from build123d import *

# Parameters (mm, degrees)
F0_W      = 498.475
F0_H      = 254
F1_DEPTH  = 36.576
F2_W      = 577.8754
F2_H      = 333.502
F3_DEPTH  = 3.175
F4_W      = 76.2
F4_H      = 114.3
F5_DEPTH  = 3.175
F6_W      = 76.2
F6_H      = 228.6
F7_DEPTH  = 3.175
F8_W      = 25.4
F8_H      = 152.4
F9_DEPTH  = 6.35
F10_W     = 25.4
F10_H     = 152.4
F11_DEPTH = 6.35
F12_W     = 571.5
F12_H     = 92.075
F13_DEPTH = 3.175
F14_W     = 508
F14_H     = 25.4
F15_DEPTH = 6.35


with BuildPart() as f1:
    # F0 (on Front) → F1 (new body)
    with BuildSketch(Plane.XZ):
        Rectangle(F0_W, F0_H)
    extrude(amount=F1_DEPTH)

    # F2 (on face) → F3 (join)
    with BuildSketch(Plane.XZ.offset(36.576)):
        Rectangle(F2_W, F2_H)
    extrude(amount=F3_DEPTH)

    # F4 (on face) → F5 (join)
    with BuildSketch(Plane.YZ.offset(288.9377)):
        with Locations((-1.651, 57.15)):
            Rectangle(F4_W, F4_H)
        with Locations((-1.651, -57.15)):
            Rectangle(F4_W, F4_H)
    extrude(amount=F5_DEPTH)

    # F6 (on face) → F7 (join)
    with BuildSketch(Plane(origin=(-288.9377, 0, 0), x_dir=(0, -1, 0), z_dir=(-1, 0, 0))):
        with Locations((1.651, 0)):
            Rectangle(F6_W, F6_H)
    extrude(amount=F7_DEPTH)

    # F8 (on face) → F9 (join)
    with BuildSketch(Plane.YZ.offset(-288.9377)):
        with Locations((-1.651, 0)):
            Rectangle(F8_W, F8_H)
    extrude(amount=F9_DEPTH)

    # F10 (on face) → F11 (join)
    with BuildSketch(Plane(origin=(288.9377, 0, 0), x_dir=(0, -1, 0), z_dir=(-1, 0, 0))):
        with Locations((1.651, 0)):
            Rectangle(F10_W, F10_H)
    extrude(amount=F11_DEPTH)

    # F12 (on face) → F13 (join)
    with BuildSketch(Plane.XY.offset(166.751)):
        with Locations((0, 6.2865)):
            Rectangle(F12_W, F12_H)
    extrude(amount=F13_DEPTH)

    # F14 (on face) → F15 (join)
    with BuildSketch(Plane(origin=(0, 0, 166.751), x_dir=(1, 0, 0), z_dir=(0, 0, -1))):
        with Locations((0, -26.924)):
            Rectangle(F14_W, F14_H)
    extrude(amount=F15_DEPTH)


solid = f1.part
Source: CAD feature listing. Evaluate the final solid. Frame: model axes, mm. A direction names the side the tool comes from. Coordinates: 2 decimals unless noted, no trailing zeros. Order: outer loops, then holes, each group sorted by start corner. A loop starts at its lowest first (then second) coordinate and runs counter-clockwise, first axis right, second up. Notation, with made-up numbers: M 5,10.25 L 25,10.25 A19 ccw 25,21.25 Z; hole C 14,-18 d11. An arc over 180 degrees is marked long. Write each question's results on one line, items separated by ' | '. Start each with the question number.
1. Section C-C, the plane x = -117. Return the cut outline in (y, z), then the cut area to 3 significant figures.
2. Section A-A, the plane y = 20.5. Return the cut outline in (x, z), then the cut area to 3 significant figures.
3. Material intervals for L1, parallel to X at y = -35, z = 31.5; L2, parallel to X at y = -5.5, z = -24; L3, parallel to Z at x = -109, y = -16, sorted ascending.
4. Section B-B, the plane z = -85. Return the cut outline in (x, y), then the cut area to 3 significant figures.
5. Draft query along Y for faces 1 (the face through (-4, -1, 166.751)), 2 (the face through (-4, -39.751, -1)), 3 (the face through (-4, 7, 169.926)). Return one class per face: +Y half, -Y half, draft (parallel to the pull), parting line (faces both ways), or undercut.
6. Section D-D, the plane z = -136. Return the cut outline in (x, y).
7. Reachability of faces 4 (the face through (-3, -18, 127)), 5 (the face through (-4, 27, 160.401)), 6 (the face through (-3, 0, 2)) from +Z, -Z, +X, -X, +Y, -Y: full face, straight path, thin tool, end or side. Return the list, or none.
8. Pin query (flat end, axial travel): pin 1 (1.6 mm diameter, centred on x = 287.5, y = -38, fed in from +Z); pin 2 (3 mm diameter, centred on x = 285.5, y = 1.5, fed in from -Z); pin 3 (7 mm diameter, centred on x = -286.5, y = 4.5, fed in from +Z); pin 4 (3 mm diameter, centred on x = -199.5, y = 24, fed in from -Z). Return the tip coordinate at first contact, or that it passes through.
Solution:
1) outline: M -39.75,-166.75 L -36.58,-166.75 L -36.58,-127 L 0,-127 L 0,127 L -36.58,127 L -36.58,166.75 L 14.22,166.75 L 14.22,160.4 L 39.62,160.4 L 39.62,166.75 L 52.32,166.75 L 52.32,169.93 L -39.75,169.93 Z | area: 10,800 mm²
2) outline: M -292.11,-114.3 L -288.94,-114.3 L -288.94,114.3 L -292.11,114.3 Z; M -285.75,166.75 L -254,166.75 L -254,160.4 L 254,160.4 L 254,166.75 L 285.75,166.75 L 285.75,169.93 L -285.75,169.93 Z; M 288.94,-114.3 L 292.11,-114.3 L 292.11,114.3 L 288.94,114.3 Z | area: 6,490 mm²
3) L1: -292.11 to -288.94, -249.24 to 249.24, 288.94 to 292.11 | L2: -292.11 to -282.59, -249.24 to 249.24, 282.59 to 292.11 | L3: -127 to 127, 166.75 to 169.93
4) outline: M -292.11,-39.75 L 292.11,-39.75 L 292.11,36.45 L 288.94,36.45 L 288.94,-36.58 L 249.24,-36.58 L 249.24,0 L -249.24,0 L -249.24,-36.58 L -288.94,-36.58 L -288.94,36.45 L -292.11,36.45 Z | area: 20,600 mm²
5) face 1: undercut | face 2: -Y half | face 3: draft
6) outline: M -288.94,-39.75 L 288.94,-39.75 L 288.94,-36.58 L -288.94,-36.58 Z
7) face 4: +X, -X, +Y | face 5: -Z, +X, -X, +Y | face 6: -Z, +Y
8) pin 1: z = 166.75 | pin 2: z = -76.2 | pin 3: z = 169.93 | pin 4: z = 160.4
